The model under review builds one solid part; all positions refer to its coordinate system, in mm. Give positions to 0.01 mm unless a question says otherwise; leave off trailing zeros. Loops run counter-clockwise (first coordinate to the right, second up) from the corner with the lowest first, then second, coordinate; pieces in that order, holes last. Notation, with made-up numbers: M -36.5,-5.5 L 20.5,-5.5 A12 cw 20.5,6.5 Z; hole C -37.5,-5.5 d3. An arc over 180 degrees is marked long. One line per item, written item: value. Start each with the question number.
Q1. Mouldability with a two-part tool opening along X and no side actions: class faces 1 (the face through (-129, -129, 3)), 2 (the face through (-1.27, -67, 4.02)), 3 (the face through (139, -2, 3)) as released by +X, released by -X, zero draft, split by the parting line, or undercut.
Q2. We need section B-B on z = 1.25. Give the number of separate pieces and of enclosed holes in the cut face, plus the area to 3 significant figures.
Q3. To check wall thickness, follow line 1 along Y through (x, z) = (-90, 5); line 2 along X through (y, z) = (30, 0.5); line 3 along Y through (x, z) = (118, 1.6). State the ranges of each line that lie inside material, in increasing order. Write a range as from..to.
Q4. We need section A-A on y = -89. Write out the cut boundary in (x, z), plus the area to 3 significant figures.
```python
from build123d import *

# Parameters (mm, degrees)
SKETCH1_W                                       = 278
SKETCH1_H                                       = 278
BOSS_EXTRUDE1_DEPTH                             = 6.35
CHAMFER1_SIZE                                   = 20
SKETCH4_R                                       = 2.75
CUT_EXTRUDE2_DEPTH                              = 76.2
SKETCH8_R                                       = 16
CUT_EXTRUDE4_DEPTH                              = 105
CSK_FOR_M4_FLAT_HEAD_MACHINE_SCREW2_D           = 4.5
CSK_FOR_M4_FLAT_HEAD_MACHINE_SCREW2_CSINK_D     = 9.4
CSK_FOR_M4_FLAT_HEAD_MACHINE_SCREW2_CSINK_ANGLE = 90
CSK_FOR_M3_FLAT_HEAD_MACHINE_SCREW1_D           = 3.4
CSK_FOR_M3_FLAT_HEAD_MACHINE_SCREW1_CSINK_D     = 6.3
CSK_FOR_M3_FLAT_HEAD_MACHINE_SCREW1_CSINK_ANGLE = 90
CSK_FOR_M3_FLAT_HEAD_MACHINE_SCREW2_D           = 3.4
CSK_FOR_M3_FLAT_HEAD_MACHINE_SCREW2_CSINK_D     = 6.3
CSK_FOR_M3_FLAT_HEAD_MACHINE_SCREW2_CSINK_ANGLE = 90


with BuildPart() as part:
    # Sketch1 → Boss-Extrude1 (new body)
    with BuildSketch(Plane.XY):
        Rectangle(SKETCH1_W, SKETCH1_H)
    extrude(amount=BOSS_EXTRUDE1_DEPTH)

    # Chamfer1
    chamfer1_edges = [part.edges().sort_by_distance(p)[0] for p in [
        (-139, 139, 3.175),
        (139, 139, 3.175),
        (139, -139, 3.175),
        (-139, -139, 3.175),
    ]]
    chamfer(chamfer1_edges, length=CHAMFER1_SIZE)

    # Sketch4 → Cut-Extrude2 (cut)
    with BuildSketch(Plane.XY.offset(6.35)):
        with Locations((-90, 130)):
            Circle(SKETCH4_R)
        with Locations((0, 151)):
            Circle(SKETCH4_R)
        with Locations((90, 130)):
            Circle(SKETCH4_R)
        with Locations((90, -130)):
            Circle(SKETCH4_R)
        with Locations((0, -151)):
            Circle(SKETCH4_R)
        with Locations((-90, -130)):
            Circle(SKETCH4_R)
    extrude(amount=-CUT_EXTRUDE2_DEPTH, mode=Mode.SUBTRACT)

    # Sketch8 → Cut-Extrude4 (cut)
    with BuildSketch(Plane.XY.offset(6.35)):
        with Locations((0, 89)):
            Circle(SKETCH8_R)
        with Locations((0, -89)):
            Circle(SKETCH8_R)
    extrude(amount=-CUT_EXTRUDE4_DEPTH, mode=Mode.SUBTRACT)

    # CSK for M4 Flat Head Machine Screw2 (through all)
    with Locations(Plane.XY.offset(6.35)):
        with Locations((0, 109), (0, 69), (0, -69), (0, -109)):
            CounterSinkHole(CSK_FOR_M4_FLAT_HEAD_MACHINE_SCREW2_D / 2, CSK_FOR_M4_FLAT_HEAD_MACHINE_SCREW2_CSINK_D / 2, counter_sink_angle=CSK_FOR_M4_FLAT_HEAD_MACHINE_SCREW2_CSINK_ANGLE)

    # CSK for M3 Flat Head Machine Screw1 (through all)
    with Locations(Plane.XY.offset(6.35)):
        with Locations((-129, 30), (-118, 30), (-118, -30), (-129, -30), (129, -30), (118, -30), (118, 30), (129, 30)):
            CounterSinkHole(CSK_FOR_M3_FLAT_HEAD_MACHINE_SCREW1_D / 2, CSK_FOR_M3_FLAT_HEAD_MACHINE_SCREW1_CSINK_D / 2, counter_sink_angle=CSK_FOR_M3_FLAT_HEAD_MACHINE_SCREW1_CSINK_ANGLE)

    # CSK for M3 Flat Head Machine Screw2 (through all)
    with Locations(Plane.XY.offset(6.35)):
        with Locations((-46.915752442, 46.109961681)):
            csk_for_m3_flat_head_machine_screw2 = CounterSinkHole(CSK_FOR_M3_FLAT_HEAD_MACHINE_SCREW2_D / 2, CSK_FOR_M3_FLAT_HEAD_MACHINE_SCREW2_CSINK_D / 2, counter_sink_angle=CSK_FOR_M3_FLAT_HEAD_MACHINE_SCREW2_CSINK_ANGLE)

    # Sketch-Pattern1: CSK for M3 Flat Head Machine Screw2 at 3 more places
    with Locations((84.166, 0.9568, 0), (90.5, -79.5, 0), (-12.5, -79.5, 0)):
        add(csk_for_m3_flat_head_machine_screw2, mode=Mode.SUBTRACT)


solid = part.part
```
Solved:
1. face 1: released by -X
1. face 2: undercut
1. face 3: released by +X
2. separate pieces: 1
2. enclosed holes: 22
2. area: 74,600 mm2
3. line 1: -139..-132.75, -127.25..127.25, 132.75..139
3. line 2: -139..-130.7, -127.3..-119.7, -116.3..116.3, 119.7..127.3, 130.7..139
3. line 3: -139..-31.7, -28.3..28.3, 31.7..139
4. outline: M -139,0 L -16,0 L -16,6.35 L -139,6.35 Z; M 16,0 L 139,0 L 139,6.35 L 16,6.35 Z
4. area: 1,560 mm2
